Verification items for this drawing (mm, ordinates from the low corner). Coordinates: 2 decimals unless noted, no trailing zeros. Write each loop counter-clockwise with the first axis right and the second up, starting at its lowest first coordinate (ties: lowest second). Pieces come first, ordered by that corner, then holes.
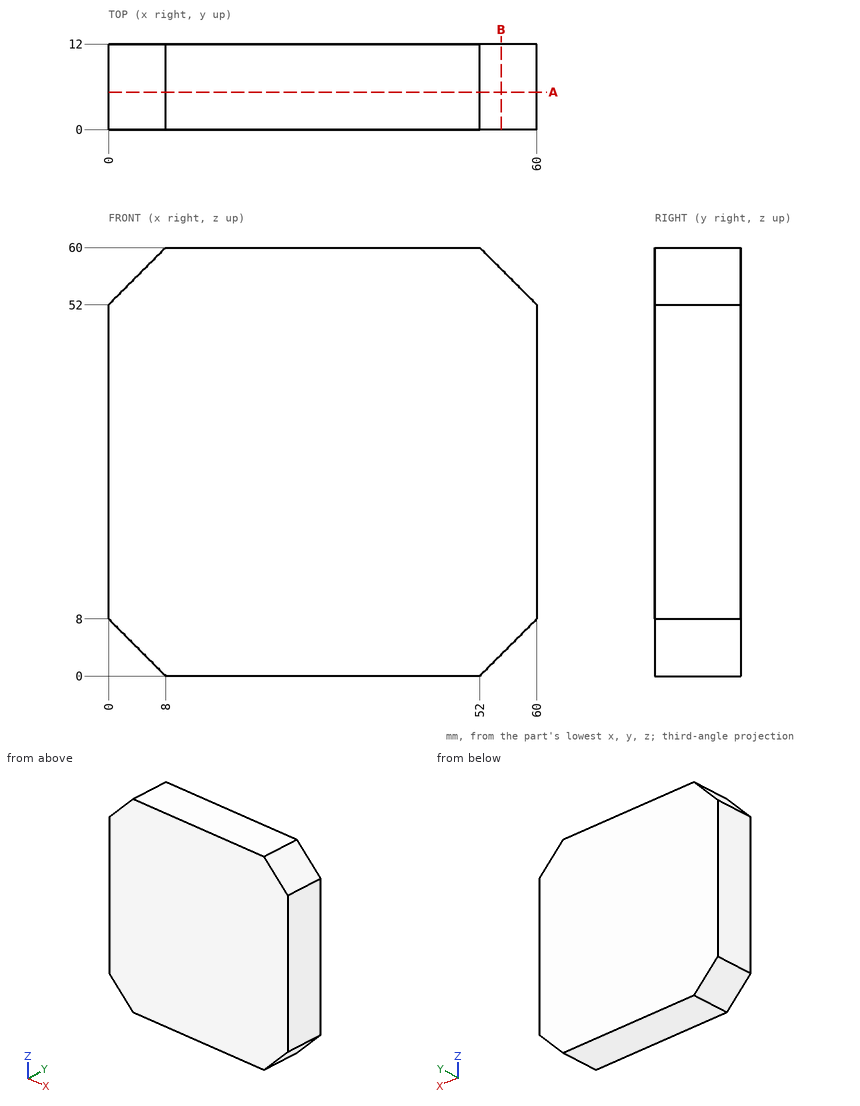
1. Sectioned sample at A-A, the plane y = 5.25. Record the boundary of the cut face in (x, z).
Computed values:
outline: (0, 8) - (8, 0) - (52, 0) - (60, 8) - (60, 52) - (52, 60) - (8, 60) - (0, 52) - close
2. Thickness scan on line 1 along X through (y, z) = (2, 53); line 2 along X through (y, z) = (4, 52.5); line 3 along Z through (x, y) = (57, 5). Record the ranges inside material, lowest first.
Computed values:
line 1: x = 1 to 59
line 2: x = 0.5 to 59.5
line 3: z = 5 to 55
3. Sectioned sample at B-B, the plane x = 55. Record the boundary of the cut face in (y, z), and give its area (3 significant figures).
Computed values:
outline: (0, 3) - (12, 3) - (12, 57) - (0, 57) - close
area: 648 mm2
